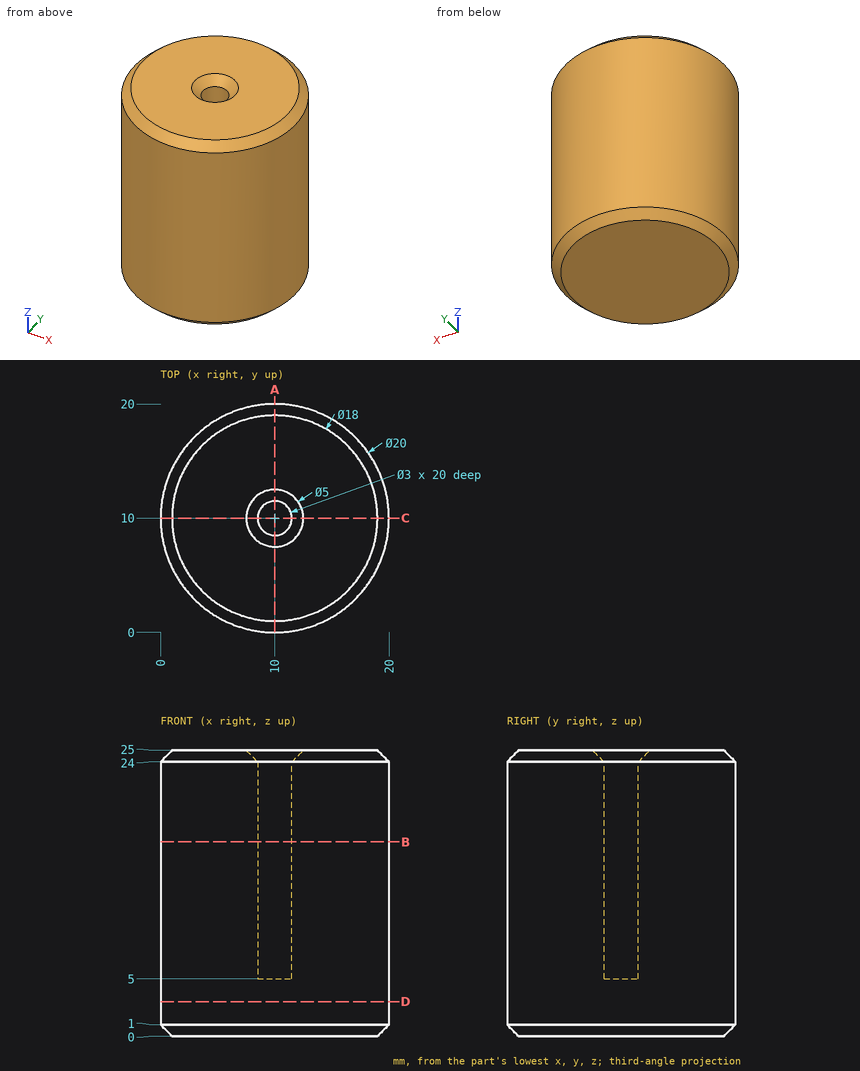
Here's the drawing with two shaded views (mm, measured from the low corner). I have some questions. Round coordinates to 2 decimals unless told otherwise and drop trailing zeros. Loops run counter-clockwise (first coordinate to the right, second up) from the corner with the lowest first, then second, coordinate; pieces in that order, holes last.
1. Suppose I cut it at A-A, the plane x = 10. Please give me the cut outline in (y, z).
Answers:
outline: (0, 1) - (1, 0) - (19, 0) - (20, 1) - (20, 24) - (19, 25) - (12.5, 25) - (11.5, 24) - (11.5, 5) - (8.5, 5) - (8.5, 24) - (7.5, 25) - (1, 25) - (0, 24) - close
2. Suppose I cut it at D-D, the plane z = 3. Please give me the cut outline in (x, y), and give its area (3 significant figures).
Answers:
outline: circle Ø20 at (10, 10)
area: 314 mm2
3. Suppose I cut it at B-B, the plane z = 17. Please give me the cut outline in (x, y).
Answers:
outline: circle Ø20 at (10, 10); hole circle Ø3 at (10, 10)
4. If I drill on probe 1 along Y at (x, z) = (10, 15); probe 2 along X at (y, z) = (10.5, 20.75); probe 3 along Y at (x, z) = (17.5, 23.5), over which ranges is the centre line in solid material (lowest first)?
Answers:
probe 1: y = 0 to 8.5, 11.5 to 20
probe 2: x = 0.01 to 8.59, 11.41 to 19.99
probe 3: y = 3.39 to 16.61
5. Will these pins go through, and if not, where does the flat tip stop? pin 1 (10 mm diameter, centred on x = 3, z = 20.5, fed in from +Y); pin 2 (1.5 mm diameter, centred on x = 10, y = 10, fed in from +Z); pin 3 (5 mm diameter, centred on y = 14, z = 4, fed in from -X).
Answers:
pin 1: stops at y = 19.8
pin 2: stops at z = 5
pin 3: stops at x = 0.11
